from build123d import *

# Parameters (mm, degrees)
SKETCH1_W           = 80
SKETCH1_H           = 5
BOSS_EXTRUDE1_DEPTH = 5
BOSS_EXTRUDE4_START = 3.5
SKETCH7_W           = 14
SKETCH7_H           = 9
BOSS_EXTRUDE4_DEPTH = 12
CUT_EXTRUDE5_START  = -3
SKETCH9_W           = 9
SKETCH9_H           = 9
CUT_EXTRUDE5_DEPTH  = 6
SKETCH11_R          = 1.1
CUT_EXTRUDE6_DEPTH  = 12
SKETCH16_R          = 3.5
BOSS_EXTRUDE7_DEPTH = 5
SKETCH15_R          = 1.1
CUT_EXTRUDE9_DEPTH  = 5
SKETCH18_R          = 1.05
CUT_EXTRUDE10_DEPTH = 5


with BuildPart() as part:
    # Sketch1 → Boss-Extrude1 (new body)
    with BuildSketch(Plane(origin=(0, 0, 0), x_dir=(1, 0, 0), z_dir=(0, 1, 0))):
        Rectangle(SKETCH1_W, SKETCH1_H)
    extrude(amount=BOSS_EXTRUDE1_DEPTH)

    # Sketch7 → Boss-Extrude4 (add)
    with BuildSketch(Plane(origin=(0, 5, 0), x_dir=(1, 0, 0), z_dir=(0, 1, 0)).offset(BOSS_EXTRUDE4_START)):
        with Locations((40, 0)):
            Rectangle(SKETCH7_W, SKETCH7_H)
    extrude(amount=-BOSS_EXTRUDE4_DEPTH)

    # Sketch9 → Cut-Extrude5 (cut)
    with BuildSketch(Plane(origin=(0, 8.5, 0), x_dir=(1, 0, 0), z_dir=(0, 1, 0)).offset(CUT_EXTRUDE5_START)):
        with Locations((42.5, 0)):
            Rectangle(SKETCH9_W, SKETCH9_H)
    extrude(amount=-CUT_EXTRUDE5_DEPTH, mode=Mode.SUBTRACT)

    # Sketch11 → Cut-Extrude6 (cut)
    with BuildSketch(Plane(origin=(0, 8.5, 0), x_dir=(1, 0, 0), z_dir=(0, 1, 0))):
        with Locations(Location((43.5, 0, 0), (0, 0, 270))):
            Circle(SKETCH11_R)
    extrude(amount=-CUT_EXTRUDE6_DEPTH, mode=Mode.SUBTRACT)

    # Sketch16 → Boss-Extrude7 (add)
    with BuildSketch(Plane(origin=(0, 5, 0), x_dir=(1, 0, 0), z_dir=(0, 1, 0))):
        with Locations((-40, 0)):
            Circle(SKETCH16_R)
    extrude(amount=-BOSS_EXTRUDE7_DEPTH)

    # Sketch15 → Cut-Extrude9 (cut)
    with BuildSketch(Plane(origin=(0, 5, 0), x_dir=(1, 0, 0), z_dir=(0, 1, 0))):
        with Locations(Location((-40, 0, 0), (0, 0, 270))):
            Circle(SKETCH15_R)
    extrude(amount=-CUT_EXTRUDE9_DEPTH, mode=Mode.SUBTRACT)

    # Sketch18 → Cut-Extrude10 (cut)
    with BuildSketch(Plane.XY.offset(2.5)):
        with Locations((-20.525255129, 2.5)):
            Circle(SKETCH18_R)
        with Locations((23.5, 2.5)):
            Circle(SKETCH18_R)
        with Locations((-25.525255129, 2.5)):
            Circle(SKETCH18_R)
        with Locations((-15.525255129, 2.5)):
            Circle(SKETCH18_R)
        with Locations((18.5, 2.5)):
            Circle(SKETCH18_R)
        with Locations((28.5, 2.5)):
            Circle(SKETCH18_R)
    extrude(amount=-CUT_EXTRUDE10_DEPTH, mode=Mode.SUBTRACT)


solid = part.part
Design review of the part built by this model. Coordinates are the model's own, in mm. A direction names the side the tool comes from. Round coordinates to 2 decimals unless told otherwise and drop trailing zeros. Loops run counter-clockwise (first coordinate to the right, second up) from the corner with the lowest first, then second, coordinate; pieces in that order, holes last. Notation, with made-up numbers: M 76,76 L 100,76 A31 ccw 100,100 Z; hole C 41.25,87 d6. An arc over 180 degrees is marked long. Answer as a JSON object with one key per item and string values.
Item 1: We need section D-D on y = -2.25. Give the boundary of the cut face in (x, z).
Answer sheet:
{"outline": "M 33,-4.5 L 47,-4.5 L 47,4.5 L 33,4.5 Z; hole C 43.5,0 d2.2"}
Item 2: We need section A-A on z = 0. State how many separate pieces and enclosed holes the cut face has, and give its area (3 significant figures).
Answer sheet:
{"separate pieces": "4", "enclosed holes": "6", "area": "452 mm^2"}
Item 3: Clearance check with flat-ended pins moving along their axes: P1, Ø2.5, axis at y = 1.5, z = 1.5, coming from the -X side; P2, Ø2.5, axis at x = -25.53, y = 2.5, coming from the -Z side; P3, Ø5, axis at x = 19.5, z = -2.5, coming from the -Y side; P4, Ø1.8, axis at x = 43.5, z = 0, coming from the +Y side. State where each tip first meets the part, or that it passes through.
Answer sheet:
{"P1": "stops at x = -43.49", "P2": "stops at z = -2.5", "P3": "stops at y = 0", "P4": "passes through"}
Item 4: Wall thickness on L1, parallel to Y at x = 23.5, z = -1.05; L2, parallel to X at y = 6.7, z = 0; L3, parallel to X at y = 6.75, z = -3: over which ranges is each line inside the solid? List them lowest first. Write a range as from..to.
Answer sheet:
{"L1": "y = 0..1.45, 3.55..5", "L2": "x = 33..42.4, 44.6..47", "L3": "x = 33..47"}
Item 5: The part is to be moulded in two halves that separate along X. For faces 1 (the flat face through (47, -2, 0)), 2 (the cylindrical face through (-43.5, 2.5, -0.1)), 3 (the cylindrical face through (29.5, 2.82, 0.04)), 4 (the flat face through (37, 3, 4.5)), say which applies: pulls with the +X half, pulls with the -X half, needs draft (parallel to the pull), parting line crosses it, or undercut.
Answer sheet:
{"face 1": "pulls with the +X half", "face 2": "undercut", "face 3": "undercut", "face 4": "needs draft"}
Item 6: We need section B-B on x = 41. Give the boundary of the cut face in (y, z), and give its area (3 significant figures).
Answer sheet:
{"outline": "M -3.5,-4.5 L -0.5,-4.5 L -0.5,4.5 L -3.5,4.5 Z; M 5.5,-4.5 L 8.5,-4.5 L 8.5,4.5 L 5.5,4.5 Z", "area": "54.0 mm^2"}
Item 7: Machinability: for faces 5 (the flat face through (-6, 5, 0)), 6 (the flat face through (38, 3, 0)), 7 (the flat face through (-3, 2, -2.5)), which of the approach directions +Z, -Z, +X, -X, +Y, -Y give a long, thin tool a straight path to every point of the face, cutting with its end or side? Answer none if there is none.
Answer sheet:
{"face 5": "+Z, -Z, -X, +Y", "face 6": "+Z, -Z, +X", "face 7": "-Z, +Y, -Y"}
